Model file for the job. Use its own axes, mm. A direction names the side the tool comes from. Round coordinates to 2 decimals unless told otherwise and drop trailing zeros. Loops run counter-clockwise (first coordinate to the right, second up) from the corner with the lowest first, then second, coordinate; pieces in that order, holes last. Notation, with made-up numbers: M -23,-0.75 L 25,-0.75 A23 cw 25,17.25 Z; hole C 25,-6 d3. An arc over 180 degrees is marked long. Answer in a Markdown table with one row per item.
from build123d import *

# Parameters (mm, degrees)
BLANKSKE_W          = 24
BLANKSKE_H          = 6.3
BLANK_DEPTH         = 2.8
TOOTHCUTSIM_DEPTH   = 25.970582692
TEETHCUTS_COUNT     = 5
TEETHCUTS_PITCH     = 6.2831853
SKETCH_1_W          = 1.366995594
SKETCH_1_H          = 6.3
SKETCH_1_W_2        = 2.499736794
CUT_EXTRUDE_1_DEPTH = 25.970582692


with BuildPart() as part:
    # BlankSke → Blank (new body)
    with BuildSketch(Plane.XY):
        with Locations((12, 3.15)):
            Rectangle(BLANKSKE_W, BLANKSKE_H)
    extrude(amount=-BLANK_DEPTH)

    # TooCutSkeSim → ToothCutSim (cut, through all)
    with BuildSketch(Plane.XY):
        Polygon((0.861870739, 1.8), (-0.861870739, 1.8), (-2.508981637, 6.3254), (2.508981637, 6.3254), align=None)
    toothcutsim = extrude(amount=-TOOTHCUTSIM_DEPTH, mode=Mode.SUBTRACT)

    # TeethCuts: ToothCutSim ×5
    with Locations(*[(i * TEETHCUTS_PITCH, 0, 0) for i in range(1, TEETHCUTS_COUNT)]):
        add(toothcutsim, mode=Mode.SUBTRACT)

    # ｽｹｯﾁ1 → ｶｯﾄ - 押し出し1 (cut, through all)
    with BuildSketch(Plane.XY):
        with Locations((23.316502203, 3.15)):
            Rectangle(SKETCH_1_W, SKETCH_1_H)
        with Locations((1.249868397, 3.15)):
            Rectangle(SKETCH_1_W_2, SKETCH_1_H)
    extrude(amount=-CUT_EXTRUDE_1_DEPTH, mode=Mode.SUBTRACT)


solid = part.part
1. Wall check: probe 1 along X at (y, z) = (4, -1.3); probe 2 along X at (y, z) = (5, -1.65). Give the ranges that are in metal, low to high.
Verdict:
| item | result |
|---|---|
| probe 1 | x = 2.5 to 4.62, 7.95 to 10.9, 14.23 to 17.19, 20.51 to 22.63 |
| probe 2 | x = 2.5 to 4.26, 8.31 to 10.54, 14.59 to 16.82, 20.88 to 22.63 |
2. Saw through at D-D (y = 4). Write the cut outline in (x, z).
Verdict:
| item | result |
|---|---|
| outline | M 2.5,-2.8 L 4.62,-2.8 L 4.62,0 L 2.5,0 Z; M 7.95,-2.8 L 10.9,-2.8 L 10.9,0 L 7.95,0 Z; M 14.23,-2.8 L 17.19,-2.8 L 17.19,0 L 14.23,0 Z; M 20.51,-2.8 L 22.63,-2.8 L 22.63,0 L 20.51,0 Z |
3. Tool access for faces 1 (the flat face through (22, 6.3, -1)), 2 (the flat face through (4.614, 4.019, -1.38)): list every direction of +Z, -Z, +X, -X, +Y, -Y with a clear straight run to the whole face (end or side of a thin tool).
Verdict:
| item | result |
|---|---|
| face 1 | +Z, -Z, +X, -X, +Y |
| face 2 | +Z, -Z, +Y |
4. Saw through at B-B (z = -2.1). Write the cut outline in (x, y).
Verdict:
| item | result |
|---|---|
| outline | M 2.5,0 L 22.63,0 L 22.63,6.3 L 21.35,6.3 L 19.71,1.8 L 17.99,1.8 L 16.35,6.3 L 15.07,6.3 L 13.43,1.8 L 11.7,1.8 L 10.07,6.3 L 8.78,6.3 L 7.15,1.8 L 5.42,1.8 L 3.78,6.3 L 2.5,6.3 Z |
5. Saw through at C-C (x = 6.25). Write the cut outline in (y, z), and give its area (3 significant figures).
Verdict:
| item | result |
|---|---|
| outline | M 0,-2.8 L 1.8,-2.8 L 1.8,0 L 0,0 Z |
| area | 5.04 mm² |
6. Saw through at A-A (y = 2.75). Write the cut outline in (x, z).
Verdict:
| item | result |
|---|---|
| outline | M 2.5,-2.8 L 5.08,-2.8 L 5.08,0 L 2.5,0 Z; M 7.49,-2.8 L 11.36,-2.8 L 11.36,0 L 7.49,0 Z; M 13.77,-2.8 L 17.64,-2.8 L 17.64,0 L 13.77,0 Z; M 20.06,-2.8 L 22.63,-2.8 L 22.63,0 L 20.06,0 Z |
7. Mould opens along X. For faces 3 (the flat face through (12, 1, 0)), 4 (the flat face through (10.897, 4.019, -1.38)), 5 (the flat face through (17.18, 4.02, -1.38)), 6 (the flat face through (2.5, 3, -1)) say: +X half, -X half, draft (parallel to the pull), parting line (faces both ways), or undercut.
Verdict:
| item | result |
|---|---|
| face 3 | draft |
| face 4 | undercut |
| face 5 | undercut |
| face 6 | -X half |
8. Pin check, flat tip, straight feed: pin 1 (0.9 mm diameter, centred on x = 18.5, z = -1, fed in from +Y). Stop position of the tip, or through.
Verdict:
| item | result |
|---|---|
| pin 1 | stops at y = 1.8 |
